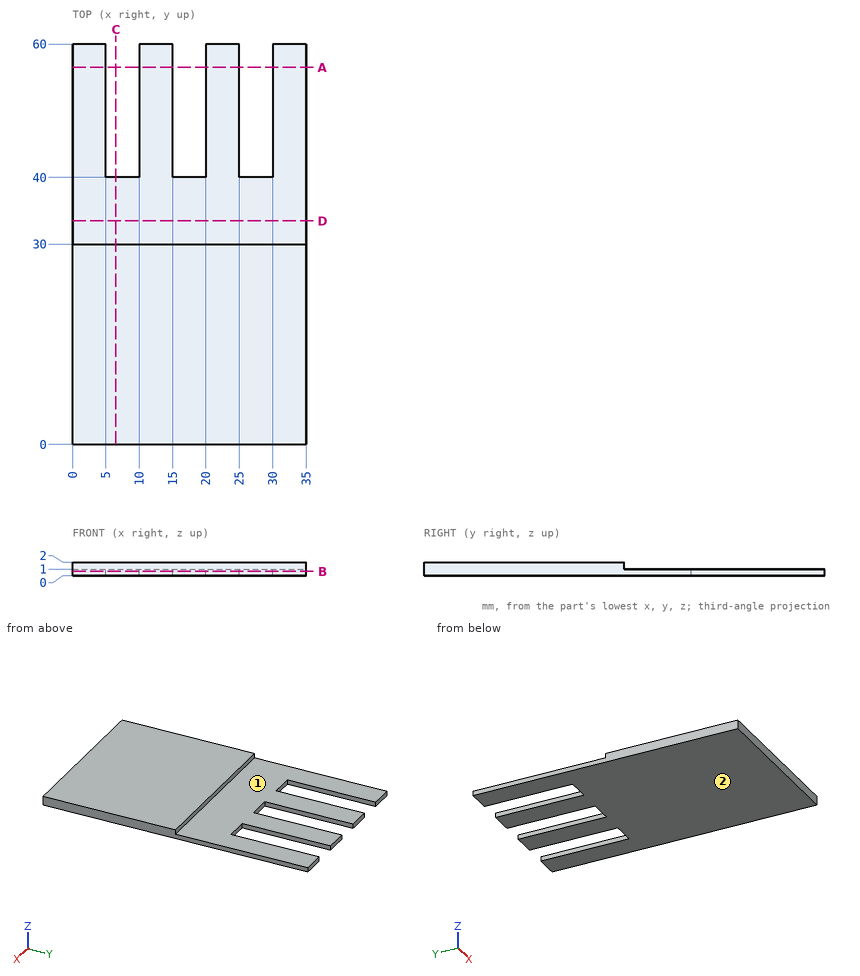
Check sheet for the drawn part. Datum: minimum x, y, z corner. Units: mm. A direction names the side the tool comes from. Round coordinates to 2 decimals unless told otherwise and drop trailing zeros. Order: outer loops, then holes, each group sorted by start corner. A loop starts at its lowest first (then second) coordinate and runs counter-clockwise, first axis right, second up. Notation, with made-up numbers: (-5, 53) - (26, 53) arc R25 ccw to (26, 73) - close; hole circle Ø4 at (68, 85). An arc over 180 degrees is marked (long way). Use a Markdown table: item, result. Add a question column.
(1) Sectioned sample at D-D, the plane y = 33.5. Enter the section's corners in (x, z).
(2) Depth check by flat-ended pin: pin 1 (0.8 mm diameter, centred on x = 24.5, z = 1.5, fed in from +Y); pin 2 (0.5 mm diameter, centred on x = 18.5, z = 0.5, fed in from +Y); pin 3 (5 mm diameter, centred on x = 22, y = 50, fed in from +Z). Enter the tip coordinate at first touch or a pass-through.
(3) Sectioned sample at B-B, the plane z = 0.65. Enter the section's corners in (x, y), and give its area (3 significant figures).
(4) Sectioned sample at A-A, the plane y = 56.5. Enter the section's corners in (x, z).
(5) Sectioned sample at C-C, the plane x = 6.5. Enter the section's corners in (y, z), and give its area (3 significant figures).
(6) Material ranges on line 1 along X through (y, z) = (43.5, 0.8); line 2 along Y through (x, z) = (26, 0.65); line 3 along Z through (x, y) = (20.5, 48), recorded low to high. Write a range as [from, to].
(7) Tool access check on the marked faces 1 and 2. Record the directions out of +Z, -Z, +X, -X, +Y, -Y that give a thin tool (end or side, any length) a straight path to the whole face; none if there is none.
Answers below:
| question | item | result |
|---|---|---|
| 1 | outline | (0, 0) - (35, 0) - (35, 1) - (0, 1) - close |
| 2 | pin 1 | y = 30 |
| 2 | pin 2 | y = 40 |
| 2 | pin 3 | z = 1 |
| 3 | outline | (0, 0) - (35, 0) - (35, 60) - (30, 60) - (30, 40) - (25, 40) - (25, 60) - (20, 60) - (20, 40) - (15, 40) - (15, 60) - (10, 60) - (10, 40) - (5, 40) - (5, 60) - (0, 60) - close |
| 3 | area | 1,800 mm² |
| 4 | outline | (0, 0) - (5, 0) - (5, 1) - (0, 1) - close; (10, 0) - (15, 0) - (15, 1) - (10, 1) - close; (20, 0) - (25, 0) - (25, 1) - (20, 1) - close; (30, 0) - (35, 0) - (35, 1) - (30, 1) - close |
| 5 | outline | (0, 0) - (40, 0) - (40, 1) - (30, 1) - (30, 2) - (0, 2) - close |
| 5 | area | 70.0 mm² |
| 6 | line 1 | [0, 5], [10, 15], [20, 25], [30, 35] |
| 6 | line 2 | [0, 40] |
| 6 | line 3 | [0, 1] |
| 7 | face 1 | +Z, +X, -X, +Y |
| 7 | face 2 | -Z, +X, -X, +Y, -Y |
